CAD build for the part. Positions are in the model's coordinates, mm. Give positions to 0.01 mm unless a question says otherwise; leave off trailing zeros. Write each loop counter-clockwise with the first axis right and the second up, starting at its lowest first coordinate (ties: lowest second). Pieces come first, ordered by that corner, then holes. Notation, with made-up numbers: (54.5, 24.5) -> (104.5, 24.5) arc R13 cw to (104.5, 49.5) -> close; hole circle Ø4 at (33.25, 84). An arc over 180 degrees is marked (long way). Answer as a JSON object with one key per item and string values.
```python
from build123d import *

# Parameters (mm, degrees)
F0_W     = 242
F0_H     = 214
F0_R     = 6.7
F1_DEPTH = 3


with BuildPart() as f1:
    # F0 (on Front) → F1 (new body)
    with BuildSketch(Plane.XZ):
        Polygon((0, -138), (0, 0), (-121, 0), (-242, 0), (-242, -138), align=None)
        with BuildLine():
            ThreePointArc((-200.3, -123), (-211.7376154339, -127.7376154339), (-207, -116.3))
            ThreePointArc((-207, -116.3), (-202.2623845661, -118.2623845661), (-200.3, -123))
        make_face(mode=Mode.SUBTRACT)
        with BuildLine():
            ThreePointArc((-207, -29.7), (-211.7376154339, -18.2623845661), (-200.3, -23))
            ThreePointArc((-200.3, -23), (-202.2623845661, -27.7376154339), (-207, -29.7))
        make_face(mode=Mode.SUBTRACT)
        with BuildLine():
            ThreePointArc((-28.3, -123), (-35, -129.7), (-41.7, -123))
            ThreePointArc((-41.7, -123), (-35, -116.3), (-28.3, -123))
        make_face(mode=Mode.SUBTRACT)
        with BuildLine():
            ThreePointArc((-28.3, -23), (-35, -29.7), (-41.7, -23))
            ThreePointArc((-41.7, -23), (-35, -16.3), (-28.3, -23))
        make_face(mode=Mode.SUBTRACT)
        with Locations((-121, -245)):
            Rectangle(F0_W, F0_H)
        Polygon((22, -138), (0, -138), (0, -352), (138, -352), (138, -138), align=None)
        with Locations((22, -313)):
            Circle(F0_R, mode=Mode.SUBTRACT)
        with BuildLine():
            ThreePointArc((115.3, -313), (117.2623845661, -308.2623845661), (122, -306.3))
            ThreePointArc((122, -306.3), (126.7376154339, -308.2623845661), (128.7, -313))
            ThreePointArc((128.7, -313), (122, -319.7), (115.3, -313))
        make_face(mode=Mode.SUBTRACT)
        with BuildLine():
            ThreePointArc((28.7, -173), (17.2623845661, -177.7376154339), (22, -166.3))
            ThreePointArc((22, -166.3), (26.7376154339, -168.2623845661), (28.7, -173))
        make_face(mode=Mode.SUBTRACT)
        with BuildLine():
            ThreePointArc((122, -179.7), (117.2623845661, -177.7376154339), (115.3, -173))
            ThreePointArc((115.3, -173), (122, -166.3), (128.7, -173))
            ThreePointArc((128.7, -173), (126.7376154339, -177.7376154339), (122, -179.7))
        make_face(mode=Mode.SUBTRACT)
        Polygon((-242, -352), (-242, -138), (-264, -138), (-380, -138), (-380, -352), align=None)
        with BuildLine():
            ThreePointArc((-357.3, -313), (-368.7376154339, -317.7376154339), (-364, -306.3))
            ThreePointArc((-364, -306.3), (-359.2623845661, -308.2623845661), (-357.3, -313))
        make_face(mode=Mode.SUBTRACT)
        with BuildLine():
            ThreePointArc((-257.3, -313), (-264, -319.7), (-270.7, -313))
            ThreePointArc((-270.7, -313), (-264, -306.3), (-257.3, -313))
        make_face(mode=Mode.SUBTRACT)
        with BuildLine():
            ThreePointArc((-364, -179.7), (-368.7376154339, -168.2623845661), (-357.3, -173))
            ThreePointArc((-357.3, -173), (-359.2623845661, -177.7376154339), (-364, -179.7))
        make_face(mode=Mode.SUBTRACT)
        with BuildLine():
            ThreePointArc((-270.7, -173), (-268.7376154339, -168.2623845661), (-264, -166.3))
            ThreePointArc((-264, -166.3), (-259.2623845661, -168.2623845661), (-257.3, -173))
            ThreePointArc((-257.3, -173), (-264, -179.7), (-270.7, -173))
        make_face(mode=Mode.SUBTRACT)
        Polygon((0, -490), (0, -352), (-242, -352), (-242, -369), (-144, -369), (-144, -473), (-242, -473), (-242, -490), (-144, -490), (-121, -490), align=None)
        with BuildLine():
            ThreePointArc((-28.3, -467), (-35, -473.7), (-41.7, -467))
            ThreePointArc((-41.7, -467), (-39.7376154339, -462.2623845661), (-35, -460.3))
            ThreePointArc((-35, -460.3), (-30.2623845661, -462.2623845661), (-28.3, -467))
        make_face(mode=Mode.SUBTRACT)
        with BuildLine():
            ThreePointArc((-28.3, -367), (-30.2623845661, -371.7376154339), (-35, -373.7))
            ThreePointArc((-35, -373.7), (-39.7376154339, -362.2623845661), (-28.3, -367))
        make_face(mode=Mode.SUBTRACT)
        Polygon((138, -138), (138, -352), (148, -352), (158, -352), (158, -138), (148, -138), align=None)
        with BuildLine():
            ThreePointArc((153, -337), (151.5355339059, -340.5355339059), (148, -342))
            ThreePointArc((148, -342), (144.4644660941, -333.4644660941), (153, -337))
        make_face(mode=Mode.SUBTRACT)
        with BuildLine():
            ThreePointArc((153, -153), (144.4644660941, -156.5355339059), (148, -148))
            ThreePointArc((148, -148), (151.5355339059, -149.4644660941), (153, -153))
        make_face(mode=Mode.SUBTRACT)
        Polygon((-390, -352), (-380, -352), (-380, -138), (-390, -138), (-400, -138), (-400, -352), align=None)
        with BuildLine():
            ThreePointArc((-385, -337), (-386.4644660941, -340.5355339059), (-390, -342))
            ThreePointArc((-390, -342), (-393.5355339059, -333.4644660941), (-385, -337))
        make_face(mode=Mode.SUBTRACT)
        with BuildLine():
            ThreePointArc((-385, -153), (-393.5355339059, -156.5355339059), (-390, -148))
            ThreePointArc((-390, -148), (-386.4644660941, -149.4644660941), (-385, -153))
        make_face(mode=Mode.SUBTRACT)
    extrude(amount=F1_DEPTH)


solid = f1.part
```
1) Pin check, flat tips, straight feed: pin 1 (1.5 mm diameter, centred on x = 86.5, y = -1.5, fed in from -Z); pin 2 (1.5 mm diameter, centred on y = -1, z = -437.5, fed in from -X); pin 3 (0.9 mm diameter, centred on y = -2, z = -38, fed in from +X). Stop position of each tip, or through.
Model answer:
{"pin 1": "stops at z = -352", "pin 2": "stops at x = -144", "pin 3": "stops at x = 0"}
2) Wall check: probe 1 along X at (y, z) = (-2.25, -313); probe 2 along X at (y, z) = (-1.65, -153); probe 3 along Z at (x, y) = (-390, -1). Give the ranges that are in metal, low to high.
Model answer:
{"probe 1": "x = -400 to -370.7, -357.3 to -270.7, -257.3 to 15.3, 28.7 to 115.3, 128.7 to 158", "probe 2": "x = -400 to -395, -385 to 143, 153 to 158", "probe 3": "z = -352 to -342, -332 to -158, -148 to -138"}
3) Slice it at C-C (z = -92.5). List the corners of the cut face in (x, y).
Model answer:
{"outline": "(-242, -3) -> (0, -3) -> (0, 0) -> (-242, 0) -> close"}
4) Mould opens along Z. For faces 1 (the cylindrical face through (-267.092, -1.479, -318.944)), 2 (the flat face through (-125, 0, -242)) say: released by +Z, released by -Z, zero draft, split by the parting line, or undercut.
Model answer:
{"face 1": "undercut", "face 2": "zero draft"}
5) Slice it at B-B (x = 95). List the corners of the cut face in (y, z), then the cut area to 3 significant figures.
Model answer:
{"outline": "(-3, -352) -> (0, -352) -> (0, -138) -> (-3, -138) -> close", "area": "642 mm2"}
6) Slice it at A-A (y = -1.75). State how many separate pieces and enclosed holes the cut face has, then the cut area to 3 significant figures.
Model answer:
{"separate pieces": "1", "enclosed holes": "18", "area": "174,000 mm2"}
